Build history of the part. All positions in model axes, mm. Round coordinates to 2 decimals unless told otherwise and drop trailing zeros. Write each loop counter-clockwise with the first axis right and the second up, starting at its lowest first coordinate (ties: lowest second). Pieces come first, ordered by that corner, then holes. Notation, with made-up numbers: M 49.25,6.25 L 72.25,6.25 A23 ccw 72.25,14.25 Z; hole C 54,-35.75 d9. An arc over 180 degrees is marked long. Write item = value, one per line. Start each with the question number.
Q1. Band-saw the part on C-C on x = 1.1. Write the cut outline in (y, z).
Q2. Band-saw the part on A-A on z = 17. Write the cut outline in (x, y), plus the area to 3 significant figures.
Q3. Band-saw the part on B-B on y = 0.75. Write the cut outline in (x, z), plus the area to 3 significant figures.
Q4. Probe L1, parallel to Z at x = 1.05, y = -0.5; L2, parallel to Z at x = 0.9, y = -6.5; L3, parallel to Y at x = 0.75, z = -17. List the from-to ranges inside material, lowest first.
Q5. Band-saw the part on D-D on y = 7. Write the cut outline in (x, z), plus the area to 3 significant figures.
Q6. Drop a flat-ended pin along its axis: P1, Ø6, axis at y = 9, z = 13, coming from the -X side. Give the stop position or say it passes through.
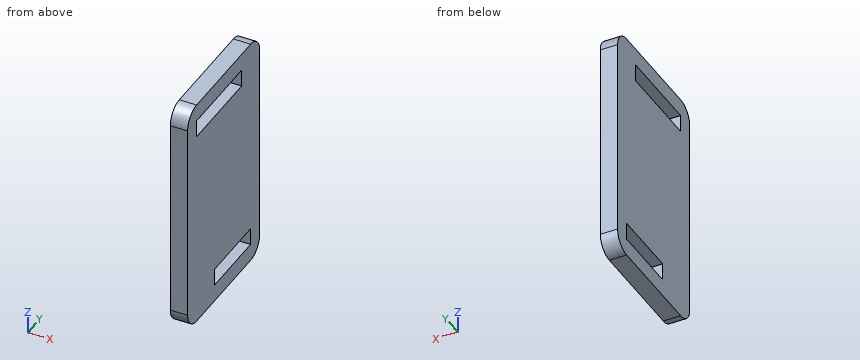
```python
from build123d import *

# Parameters (mm, degrees)
SKETCH_2_W      = 3
SKETCH_2_H      = 15
SKETCH_2_H_2    = 12
EXTRUDE_1_DEPTH = 3
FILLET_1_R      = 3


with BuildPart() as part:
    # Sketch 2 → Extrude 1 (new body)
    with BuildSketch(Plane(origin=(0, 0, 0), x_dir=(0, 0, -1), z_dir=(1, 0, 0))):
        Polygon((-20.5, -9), (-20.5, 12), (20.5, 12), (20.5, -12), (-20.5, -12), align=None)
        with Locations((-16, -1.5)):
            Rectangle(SKETCH_2_W, SKETCH_2_H, mode=Mode.SUBTRACT)
        with Locations((16, 3)):
            Rectangle(SKETCH_2_W, SKETCH_2_H_2, mode=Mode.SUBTRACT)
    extrude(amount=EXTRUDE_1_DEPTH)

    # Fillet 1
    fillet_1_edges = [part.edges().sort_by_distance(p)[0] for p in [
        (1.5, 12, 20.5),
        (1.5, 12, -20.5),
        (1.5, -12, -20.5),
        (1.5, -12, 20.5),
    ]]
    fillet(fillet_1_edges, radius=FILLET_1_R)


solid = part.part
```
Conclusion:
q1.outline = M -12,-17.5 A3 ccw -9,-20.5 L 9,-20.5 A3 ccw 12,-17.5 L 12,17.5 A3 ccw 9,20.5 L -9,20.5 A3 ccw -12,17.5 Z; hole M -9,14.5 L 6,14.5 L 6,17.5 L -9,17.5 Z; hole M -3,-17.5 L 9,-17.5 L 9,-14.5 L -3,-14.5 Z
q2.outline = M 0,-12 L 3,-12 L 3,-9 L 0,-9 Z; M 0,6 L 3,6 L 3,12 L 0,12 Z
q2.area = 27.0 mm^2
q3.outline = M 0,-20.5 L 3,-20.5 L 3,-17.5 L 0,-17.5 Z; M 0,-14.5 L 3,-14.5 L 3,14.5 L 0,14.5 Z; M 0,17.5 L 3,17.5 L 3,20.5 L 0,20.5 Z
q3.area = 105 mm^2
q4.L1 = -20.5 to -17.5, -14.5 to 14.5, 17.5 to 20.5
q4.L2 = -20.5 to 14.5, 17.5 to 20.5
q4.L3 = -12 to -3, 9 to 12
q5.outline = M 0,-20.5 L 3,-20.5 L 3,-17.5 L 0,-17.5 Z; M 0,-14.5 L 3,-14.5 L 3,20.5 L 0,20.5 Z
q5.area = 114 mm^2
q6.P1 = 0
